Can you work these out from the drawing? Everything is in mm from the part's minimum corner. A direction names the side the tool comes from. Coordinates: 2 decimals unless noted, no trailing zeros. Loops run counter-clockwise (first coordinate to the right, second up) from the corner with the lowest first, then second, coordinate; pieces in that order, holes last.
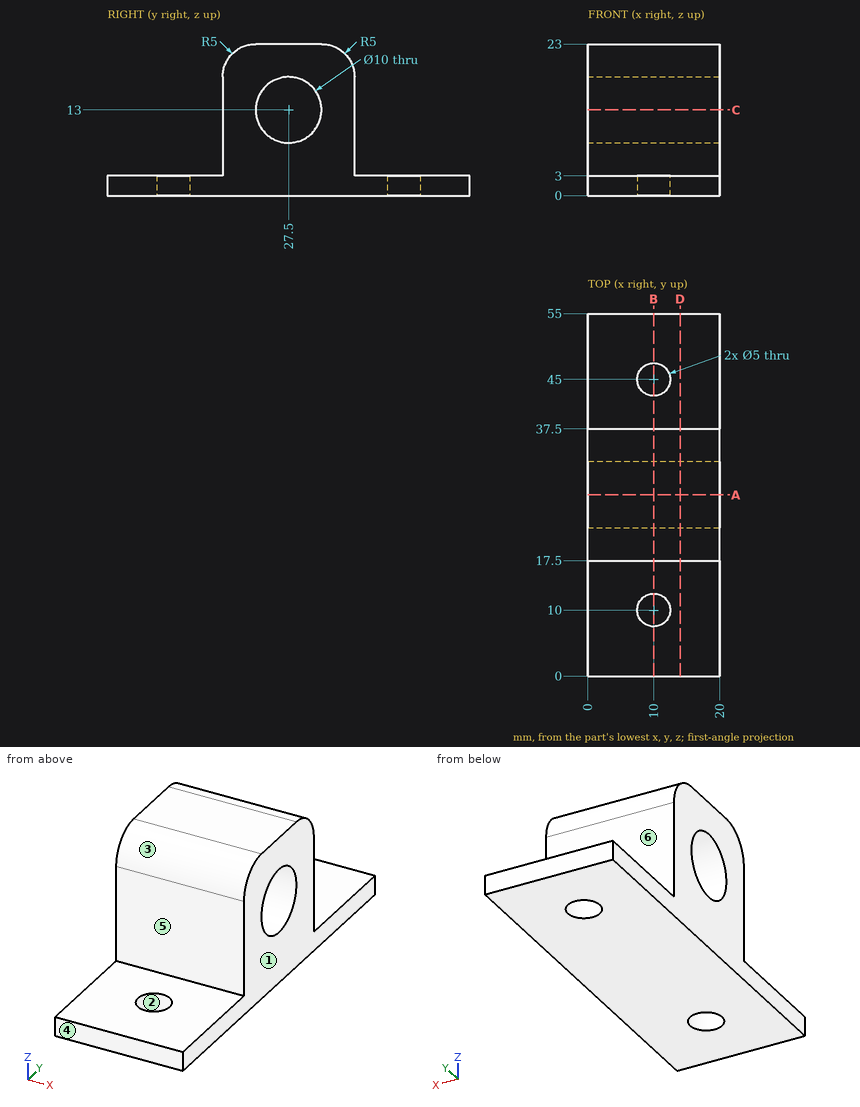
1) Imagine slicing it at C-C on z = 13. List the corners of the cut face in (x, y) for me, plus the area to 3 significant figures.
2) Imagine slicing it at A-A on y = 27.5. List the corners of the cut face in (x, z) for me.
3) For the marked faces 4, 5 and 6, which set-ups out of +Z, -Z, +X, -X, +Y, -Y let a thin tool reach every point of the face, with its end or its side?
4) If I drill on L1, parallel to Y at x = 10, z = 1.95; L2, parallel to X at y = 10, z = 0.7; L3, parallel to Z at x = 14.25, y = 27.5, over which ranges is the centre line in solid material (lowest first)?
5) Will these pins go through, and if not, where does the flat tip stop? pin 1 (2 mm diameter, centred on y = 28.5, z = 15, fed in from +X); pin 2 (6.5 mm diameter, centred on x = 10, y = 10, fed in from +Z); pin 3 (7.5 mm diameter, centred on x = 8.5, z = 13.5, fed in from -Y); pin 4 (8 mm diameter, centred on x = 8, z = 9.5, fed in from +Y).
6) We'd pull the mould along X, two halves only. Please class the marked faces 1, 2 and 3: released by +X, released by -X, zero draft, split by the parting line, or undercut.
7) Imagine slicing it at B-B on x = 10. List the corners of the cut face in (y, z) for me, plus the area to 3 significant figures.
8) Imagine slicing it at D-D on x = 14. List the corners of the cut face in (y, z) for me.
Solved:
1. outline: (0, 17.5) - (20, 17.5) - (20, 22.5) - (0, 22.5) - close; (0, 32.5) - (20, 32.5) - (20, 37.5) - (0, 37.5) - close
1. area: 200 mm2
2. outline: (0, 0) - (20, 0) - (20, 8) - (0, 8) - close; (0, 18) - (20, 18) - (20, 23) - (0, 23) - close
3. face 4: +Z, -Z, +X, -X, -Y
3. face 5: +Z, +X, -X, -Y
3. face 6: +Z, +X, -X, +Y
4. L1: y = 0 to 7.5, 12.5 to 42.5, 47.5 to 55
4. L2: x = 0 to 7.5, 12.5 to 20
4. L3: z = 0 to 8, 18 to 23
5. pin 1: passes through
5. pin 2: stops at z = 3
5. pin 3: stops at y = 17.5
5. pin 4: stops at y = 37.5
6. face 1: released by +X
6. face 2: undercut
6. face 3: zero draft
7. outline: (0, 0) - (7.5, 0) - (7.5, 3) - (0, 3) - close; (12.5, 0) - (42.5, 0) - (42.5, 3) - (37.5, 3) - (37.5, 18) arc R5 ccw to (32.5, 23) - (22.5, 23) arc R5 ccw to (17.5, 18) - (17.5, 3) - (12.5, 3) - close; (47.5, 0) - (55, 0) - (55, 3) - (47.5, 3) - close; hole circle Ø10 at (27.5, 13)
7. area: 446 mm2
8. outline: (0, 0) - (55, 0) - (55, 3) - (37.5, 3) - (37.5, 18) arc R5 ccw to (32.5, 23) - (22.5, 23) arc R5 ccw to (17.5, 18) - (17.5, 3) - (0, 3) - close; hole circle Ø10 at (27.5, 13)
